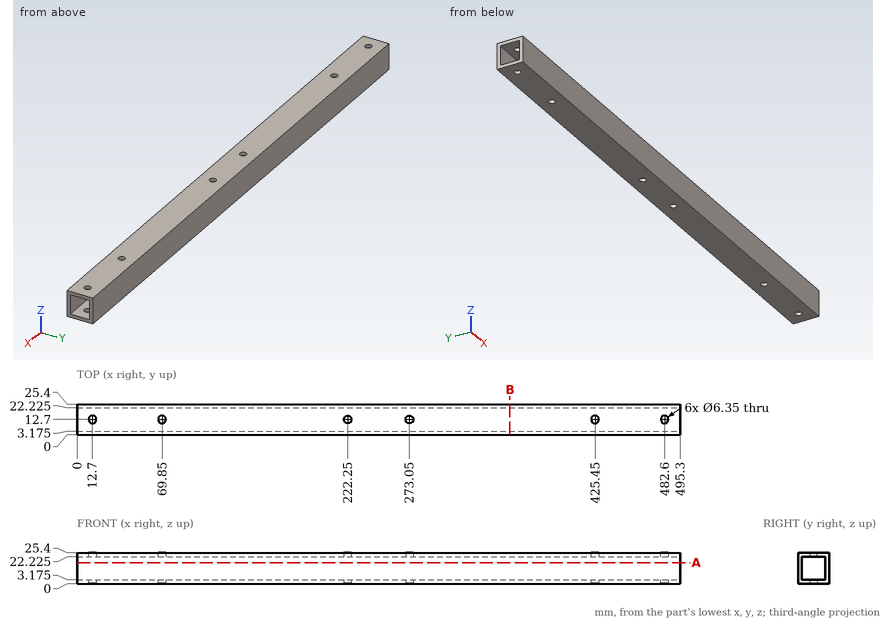
Study the drawing (mm; zero at the part's minimum x, y, z) and answer. Coordinates: 2 decimals unless noted, no trailing zeros. Loops run counter-clockwise (first coordinate to the right, second up) from the corner with the lowest first, then second, coordinate; pieces in that order, holes last. Notation, with made-up numbers: M -7.5,3 L -2.5,3 A16 cw -2.5,12 Z; hole C 42.25,18 d7. An arc over 180 degrees is marked long. Answer in a Markdown table with one row per item. Add a question column.
1. Flat-ended cylindrical pins translate along their axes: P1, Ø7.5, axis at x = 12.7, y = 12.7, coming from the -Z side; P2, Ø2, axis at y = 4.5, z = 11.5, coming from the -X side. Find the tip coordinate at first contact, or state that the pin passes through.
2. Find section A-A, the plane z = 17.5. Write down the section's boundary in (x, y) (3 decimals).
3. Find section B-B, the plane x = 355.5. Write down the section's boundary in (y, z) (3 decimals), then the cut area to 3 significant figures.
4. Consider L1, parallel to Z at x = 28, y = 11.5 (3 decimals); L2, parallel to Y at x = 482.6, z = 24.2 (3 decimals). Determine where each line is inside the solid, lowest interval first.
Reported:
| question | item | result |
|---|---|---|
| 1 | P1 | stops at z = 0 |
| 1 | P2 | passes through |
| 2 | outline | M 0,0 L 495.3,0 L 495.3,3.175 L 0,3.175 Z; M 0,22.225 L 495.3,22.225 L 495.3,25.4 L 0,25.4 Z |
| 3 | outline | M 0,0 L 25.4,0 L 25.4,25.4 L 0,25.4 Z; hole M 3.175,3.175 L 22.225,3.175 L 22.225,22.225 L 3.175,22.225 Z |
| 3 | area | 282 mm^2 |
| 4 | L1 | z = 0 to 3.175, 22.225 to 25.4 |
| 4 | L2 | y = 0 to 9.525, 15.875 to 25.4 |
